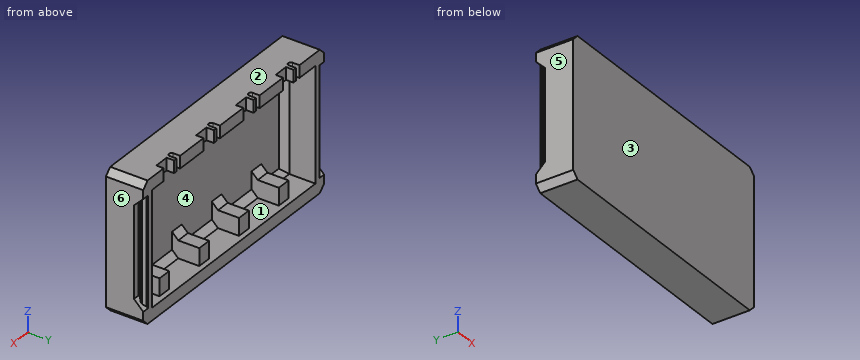
```python
from build123d import *

# Parameters (mm, degrees)
SKETCH2_W           = 210
SKETCH2_H           = 112
SKETCH2_W_2         = 190
SKETCH2_H_2         = 92
BOSS_EXTRUDE1_DEPTH = 30.16
SKETCH3_W           = 210
SKETCH3_H           = 112
BOSS_EXTRUDE2_DEPTH = 4
SKETCH4_W           = 11.25
SKETCH4_H           = 13.999999996
BOSS_EXTRUDE3_DEPTH = 22
SKETCH5_W           = 12
SKETCH5_H           = 10
CUT_EXTRUDE1_DEPTH  = 6
CHAMFER2_SIZE       = 5
CUT_EXTRUDE2_DEPTH  = 5.5
CUT_EXTRUDE3_DEPTH  = 5.5
SKETCH9_W           = 4.2
SKETCH9_H           = 10
CUT_EXTRUDE4_DEPTH  = 7.5
FILLET1_R           = 1.88
CHAMFER3_SIZE       = 5
CHAMFER4_SIZE       = 5
BOSS_EXTRUDE4_START = -10
BOSS_EXTRUDE4_DEPTH = 90


with BuildPart() as part:
    # Sketch2 → Boss-Extrude1 (new body)
    with BuildSketch(Plane(origin=(0, 0, 0), x_dir=(1, 0, 0), z_dir=(0, 1, 0))):
        with Locations((-15.529354961, -23.471700962)):
            Rectangle(SKETCH2_W, SKETCH2_H)
        with Locations((-15.529354961, -23.471700962)):
            Rectangle(SKETCH2_W_2, SKETCH2_H_2, mode=Mode.SUBTRACT)
    extrude(amount=BOSS_EXTRUDE1_DEPTH)



with BuildPart() as body_2:
    # Sketch3 → Boss-Extrude2 (new body)
    with BuildSketch(Plane.XZ):
        with Locations((-15.529354961, 23.471700962)):
            Rectangle(SKETCH3_W, SKETCH3_H)
    extrude(amount=-BOSS_EXTRUDE2_DEPTH)


with BuildPart() as part_1:
    add(part.part)

    add(body_2.part)  # Boss-Extrude3 merges body 2
    # Sketch4 → Boss-Extrude3 (add)
    with BuildSketch(Plane(origin=(0, 4, 0), x_dir=(1, 0, 0), z_dir=(0, 1, 0))):
        with Locations((-79.564354961, 15.52829904)):
            Rectangle(SKETCH4_W, SKETCH4_H)
        with Locations((-33.394354961, 15.52829904)):
            Rectangle(SKETCH4_W, SKETCH4_H)
        with Locations((12.775645039, 15.52829904)):
            Rectangle(SKETCH4_W, SKETCH4_H)
        with Locations((58.945645039, 15.52829904)):
            Rectangle(SKETCH4_W, SKETCH4_H)
    extrude(amount=BOSS_EXTRUDE3_DEPTH)

    # Sketch5 → Cut-Extrude1 (cut)
    with BuildSketch(Plane(origin=(0, 30.16, 0), x_dir=(1, 0, 0), z_dir=(0, 1, 0))):
        with Locations((-78.829354961, -74.471700962)):
            Rectangle(SKETCH5_W, SKETCH5_H)
        with Locations((-32.659354961, -74.471700962)):
            Rectangle(SKETCH5_W, SKETCH5_H)
        with Locations((13.510645039, -74.471700962)):
            Rectangle(SKETCH5_W, SKETCH5_H)
        with Locations((59.680645039, -74.471700962)):
            Rectangle(SKETCH5_W, SKETCH5_H)
    extrude(amount=-CUT_EXTRUDE1_DEPTH, mode=Mode.SUBTRACT)

    # Chamfer2
    chamfer2_edges = [part_1.edges().sort_by_distance(p)[0] for p in [
        (-110.529354961, 4, 23.471700962),
        (-97.859354961, 4, -22.528299038),
        (-56.479354961, 4, -22.528299038),
        (79.470645039, 4, 23.471700962),
        (-15.529354961, 4, 69.471700962),
        (-10.309354961, 4, -22.528299038),
        (35.860645039, 4, -22.528299038),
        (72.020645039, 4, -22.528299038),
    ]]
    chamfer(chamfer2_edges, length=CHAMFER2_SIZE)

    # Sketch6 → Cut-Extrude2 (cut)
    with BuildSketch(Plane.ZY.offset(120.529354961)):
        Polygon((-20.528299038, 30.16), (67.471700962, 30.16), (59.971700962, 22.66), (-13.028299038, 22.66), align=None)
    extrude(amount=-CUT_EXTRUDE2_DEPTH, mode=Mode.SUBTRACT)

    # Sketch8 → Cut-Extrude3 (cut)
    with BuildSketch(Plane(origin=(89.470645039, 0, 0), x_dir=(0, 0, -1), z_dir=(1, 0, 0))):
        Polygon((20.528299038, 30.16), (13.028299038, 22.66), (-59.971700962, 22.66), (-67.471700962, 30.16), align=None)
    extrude(amount=-CUT_EXTRUDE3_DEPTH, mode=Mode.SUBTRACT)

    # Sketch9 → Cut-Extrude4 (cut)
    with BuildSketch(Plane(origin=(0, 30.16, 0), x_dir=(1, 0, 0), z_dir=(0, 1, 0))):
        with Locations((-89.789354961, -74.471700962)):
            Rectangle(SKETCH9_W, SKETCH9_H)
        with Locations((48.720645039, -74.471700962)):
            Rectangle(SKETCH9_W, SKETCH9_H)
        with Locations((2.550645039, -74.471700962)):
            Rectangle(SKETCH9_W, SKETCH9_H)
        with Locations((-43.619354961, -74.471700962)):
            Rectangle(SKETCH9_W, SKETCH9_H)
    extrude(amount=-CUT_EXTRUDE4_DEPTH, mode=Mode.SUBTRACT)

    # Fillet1
    fillet1_edges = [part_1.edges().sort_by_distance(p)[0] for p in [
        (-87.689354961, 22.66, 74.471700962),
        (-91.889354961, 22.66, 74.471700962),
        (50.820645039, 22.66, 74.471700962),
        (46.620645039, 22.66, 74.471700962),
        (4.650645039, 22.66, 74.471700962),
        (0.450645039, 22.66, 74.471700962),
        (-41.519354961, 22.66, 74.471700962),
        (-45.719354961, 22.66, 74.471700962),
    ]]
    fillet(fillet1_edges, radius=FILLET1_R)

    # Chamfer3
    chamfer3_edges = [part_1.edges().sort_by_distance(p)[0] for p in [
        (-79.564354961, 4, -8.528299042),
        (-33.394354961, 4, -8.528299042),
        (12.775645039, 4, -8.528299042),
        (58.945645039, 4, -8.528299042),
    ]]
    chamfer(chamfer3_edges, length=CHAMFER3_SIZE)

    # Chamfer4
    chamfer4_edges = [part_1.edges().sort_by_distance(p)[0] for p in [
        (89.470645039, 15.08, 79.471700962),
        (-120.529354961, 15.08, 79.471700962),
        (-120.529354961, 15.08, -32.528299038),
        (89.470645039, 15.08, -32.528299038),
    ]]
    chamfer(chamfer4_edges, length=CHAMFER4_SIZE)

    # Sketch10 → Boss-Extrude4 (add)
    with BuildSketch(Plane.XY.offset(79.471700962).offset(BOSS_EXTRUDE4_START)):
        Polygon((83.970645039, 29.16), (86.220645039, 26.91), (86.220645039, 25.91), (83.970645039, 23.66), align=None)
        Polygon((-115.029354961, 29.16), (-115.029354961, 23.66), (-117.279354961, 25.91), (-117.279354961, 26.91), align=None)
    extrude(amount=-BOSS_EXTRUDE4_DEPTH)


solid = part_1.part
```
Source: CAD feature listing. Evaluate the final solid. Frame: model axes, mm. Face numbers are marked on the shaded views. A direction names the side the tool comes from. Round coordinates to 2 decimals unless told otherwise and drop trailing zeros. Write each loop counter-clockwise with the first axis right and the second up, starting at its lowest first coordinate (ties: lowest second). Pieces come first, ordered by that corner, then holes. Notation, with made-up numbers: M 34,-28 L 50,-28 A20 cw 50,4 Z; hole C 81.25,-28 d1. An arc over 180 degrees is marked long. Answer as a JSON object with one key per item and string values. Group by question number.
(1) First-contact query: pin 1 (1.5 mm diameter, centred on x = -52, z = 3, fed in from +Y); pin 2 (5 mm diameter, centred on x = 62.5, z = 76, fed in from +Y); pin 3 (1.1 mm diameter, centred on y = 30, z = 24, fed in from -X). Flat tips, straight axial feed; report the tip coordinate or a pass-through.
(2) Ray query, line 1 (Z direction, x = 38, y = 7); line 2 (X direction, y = 14, z = 67); line 3 (Z direction, x = -72.5, y = 10). Return the intervals inside material, ascending. Write a range as [from, to].
(3) Section query B-B on z = 48.5. Output: boundary loops of the cut face in (x, y), then the cut area to 3 significant figures.
(4) Section query C-C on x = 12. Output: boundary loops of the cut face in (y, z).
(5) Reachability of the marked faces 1 and 2 from +Z, -Z, +X, -X, +Y, -Y: full face, straight path, thin tool, end or side. Return the list, or none.
(6) Section query A-A on y = 11.5. Output: boundary loops of the cut face in (x, z).
(7) Mould query, pull axis X, two halves, no side actions, for the marked faces 3, 4, 5 and 6. Classes: +X half, -X half, draft (parallel to the pull), parting line (faces both ways), or undercut.
Computed values:
{
 "1": {"pin 1": "y = 4", "pin 2": "y = 24.16", "pin 3": "x = -115.03"},
 "2": {"line 1": "[-32.53, -20.53], [67.47, 79.47]", "line 2": "[-120.53, -110.53], [79.47, 89.47]", "line 3": "[-32.53, -22.53], [69.47, 79.47]"},
 "3": {"outline": "M -120.53,0 L 89.47,0 L 89.47,22.66 L 83.97,22.66 L 83.97,23.66 L 86.22,25.91 L 86.22,26.91 L 83.97,29.16 L 83.97,30.16 L 79.47,30.16 L 79.47,9 L 74.47,4 L -105.53,4 L -110.53,9 L -110.53,30.16 L -115.03,30.16 L -115.03,29.16 L -117.28,26.91 L -117.28,25.91 L -115.03,23.66 L -115.03,22.66 L -120.53,22.66 Z", "area": "1,320 mm^2"},
 "4": {"outline": "M 0,-32.53 L 30.16,-32.53 L 30.16,-22.53 L 26,-22.53 L 26,-8.53 L 9,-8.53 L 4,-3.53 L 4,64.47 L 9,69.47 L 24.16,69.47 L 24.16,79.47 L 0,79.47 Z"},
 "5": {"face 1": "+Y", "face 2": "+Z, +X, -X, +Y, -Y"},
 "6": {"outline": "M -120.53,-27.53 L -115.53,-32.53 L 84.47,-32.53 L 89.47,-27.53 L 89.47,74.47 L 84.47,79.47 L -115.53,79.47 L -120.53,74.47 Z; hole M -110.53,-22.53 L -85.19,-22.53 L -85.19,-8.53 L -73.94,-8.53 L -73.94,-22.53 L -39.02,-22.53 L -39.02,-8.53 L -27.77,-8.53 L -27.77,-22.53 L 7.15,-22.53 L 7.15,-8.53 L 18.4,-8.53 L 18.4,-22.53 L 53.32,-22.53 L 53.32,-8.53 L 64.57,-8.53 L 64.57,-22.53 L 79.47,-22.53 L 79.47,69.47 L -110.53,69.47 Z"},
 "7": {"face 3": "draft", "face 4": "undercut", "face 5": "-X half", "face 6": "+X half"}
}
